Part model, mm, in its own coordinate system. Face numbers are marked on the shaded views. A direction names the side the tool comes from. Round coordinates to 2 decimals unless told otherwise and drop trailing zeros. Loops run counter-clockwise (first coordinate to the right, second up) from the corner with the lowest first, then second, coordinate; pieces in that order, holes last. Notation, with made-up numbers: M 33,-21 L 58,-21 A16 cw 58,0 Z; hole C 1,15 d6. An arc over 180 degrees is marked long. Write each question's results on one line, items separated by ' | '.
from build123d import *

# Parameters (mm, degrees)
BOSS_EXTRUDE1_DEPTH        = 5
F_4_5_4_5_DIAMETER_HOLE1_D = 4.5
F_4_5_4_5_DIAMETER_HOLE2_D = 4.5
CHAMFER3_SIZE              = 1.737611999
CHAMFER3_SIZE2             = 3.873994542
SKETCH18_R                 = 2.25
CUT_EXTRUDE1_DEPTH         = 10


with BuildPart() as part:
    # Sketch1 → Boss-Extrude1 (new body)
    with BuildSketch(Plane.XZ.offset(73)):
        with BuildLine():
            Line((47.401706558, 28.464616212), (51.486447787, 32.952250014))
            Line((51.486447787, 32.952250014), (77.985492495, 35.143180318))
            ThreePointArc((77.985492495, 35.143180318), (87.173153133, 38.077045167), (80.988712415, 45.477948081))
            Line((80.988712415, 45.477948081), (42.966330666, 41.501731436))
            Line((42.966330666, 41.501731436), (23.877297166, 43.453769804))
            ThreePointArc((23.877297166, 43.453769804), (18.123943846, 39.278307812), (22.299405838, 33.524954492))
            Line((22.299405838, 33.524954492), (47.401706558, 28.464616212))
        make_face()
    extrude(amount=-BOSS_EXTRUDE1_DEPTH)

    # Ø4.5 (4.5) Diameter Hole1 (through all)
    with Locations(Plane(origin=(0, -73, 0), x_dir=(-1, 0, 0), z_dir=(0, -1, 0))):
        with Locations((-45.629259616, -33.33886952)):
            Hole(F_4_5_4_5_DIAMETER_HOLE1_D / 2)

    # Ø4.5 (4.5) Diameter Hole2 (through all)
    with Locations(Plane(origin=(0, -73, 0), x_dir=(-1, 0, 0), z_dir=(0, -1, 0))):
        with Locations((-22.965684709, -38.284870865)):
            Hole(F_4_5_4_5_DIAMETER_HOLE2_D / 2)

    # Chamfer3
    chamfer3_edges = [part.edges().sort_by_distance(p)[0] for p in [
        (47.401706558, -70.5, 28.464616212),
    ]]
    chamfer3_side = [part.faces().sort_by_distance(p)[0] for p in [
        (49.444077173, -70.5, 30.708433113),
    ]]
    chamfer(chamfer3_edges, length=CHAMFER3_SIZE, length2=CHAMFER3_SIZE2, reference=chamfer3_side[0])

    # Sketch18 → Cut-Extrude1 (cut)
    with BuildSketch(Plane(origin=(0, -68, 0), x_dir=(1, 0, 0), z_dir=(0, 1, 0))):
        with Locations((81.593094218, -39.698575952)):
            Circle(SKETCH18_R)
    extrude(amount=-CUT_EXTRUDE1_DEPTH, mode=Mode.SUBTRACT)


solid = part.part
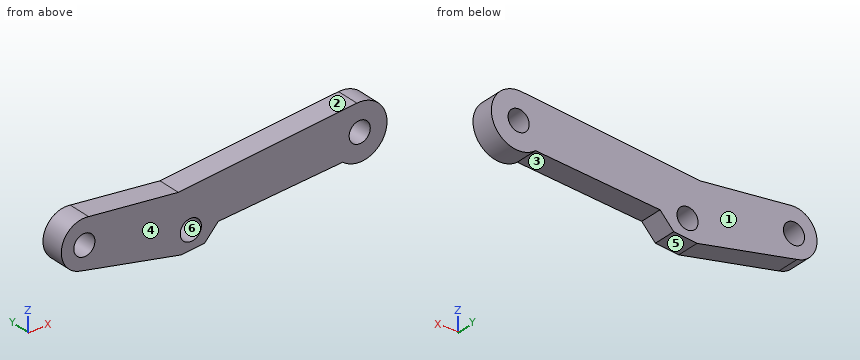
Item 1: Drop flat-ended pins along their axis: P1, Ø2.5, axis at x = 22.97, z = 38.28, coming from the +Y side; P2, Ø2, axis at x = 36.5, y = -70.5, coming from the -Z side; P3, Ø1.5, axis at x = 45.5, y = -69, coming from the -Z side; P4, Ø1.5, axis at x = 59.5, y = -71.5, coming from the -Z side. Give the stop position or say it passes through.
Filled sheet:
P1: through | P2: z = 30.46 | P3: z = 29.35 | P4: z = 33.55
Item 2: Band-saw the part on D-D on x = 30. Give the cut face in (y, z).
Filled sheet:
outline: M -73,31.97 L -68,31.97 L -68,42.83 L -73,42.83 Z
Item 3: Band-saw the part on B-B on z = 34.5. Give the cut face in (x, y).
Filled sheet:
outline: M 20.03,-73 L 43.7,-73 L 43.7,-68 L 20.03,-68 Z; M 47.56,-73 L 70.21,-73 L 70.21,-68 L 47.56,-68 Z; M 79,-73 L 84.19,-73 L 84.19,-68 L 79,-68 Z
Item 4: Two-plate mould, pull along Z, no slides. Class the marked faces 4, 5 and 6: +Z half, -Z half, draft (parallel to the pull), parting line (faces both ways), or undercut.
Filled sheet:
face 4: draft | face 5: -Z half | face 6: undercut
Item 5: Which spindle directions (+Z, -Z, +X, -X, +Y, -Y) get a long thin tool onto all of the face, cutting with end or side? Do the marked faces 1, 2 and 3. Say none if no direction does.
Filled sheet:
face 1: +Z, -Z, +X, -X, +Y | face 2: +Z, +Y, -Y | face 3: -Z, +Y, -Y
Item 6: Band-saw the part on A-A on x = 47. Give the cut face in (y, z), and give its area (3 significant figures).
Filled sheet:
outline: M -73,29.59 L -68,29.59 L -68,31.55 L -73,31.55 Z; M -73,35.12 L -68,35.12 L -68,41.92 L -73,41.92 Z | area: 43.8 mm^2
Item 7: Band-saw the part on C-C on y = -69.1. Give the cut face in (x, z), and give its area (3 significant figures).
Filled sheet:
outline: M 22.3,33.52 L 43.6,29.23 L 48.57,29.75 L 51.49,32.95 L 77.99,35.14 A5.81 ccw long 80.99,45.48 L 42.97,41.5 L 23.88,43.45 A5.03 ccw Z; hole C 22.97,38.28 d4.5; hole C 45.63,33.34 d4.5; hole C 81.59,39.7 d4.5 | area: 665 mm^2
Item 8: Wall check: L1, parallel to X at y = -69.55, z = 39.25; L2, parallel to X at y = -68.7, z = 39; L3, parallel to Z at x = 82, y = -69.45. Give the ranges that are in metal, low to high.
Filled sheet:
L1: 18.12 to 20.93, 25 to 79.39, 83.8 to 87.39 | L2: 18.09 to 20.83, 25.1 to 79.45, 83.73 to 87.36 | L3: 33.9 to 37.49, 41.91 to 45.5
